The listing builds one solid part. Answer for the finished solid, in the listing's coordinates (mm). Give positions to 0.01 mm unless a question says otherwise; leave off trailing zeros. Write each loop counter-clockwise with the first axis right and the second up, starting at its lowest first coordinate (ties: lowest second). Pieces come first, ordered by that corner, then holes.
```python
from build123d import *

# Parameters (mm, degrees)
BOSS_EXTRUDE4_DEPTH                             = 4.5
CSK_FOR_M3_FLAT_HEAD_MACHINE_SCREW1_D           = 3.4
CSK_FOR_M3_FLAT_HEAD_MACHINE_SCREW1_CSINK_D     = 6.3
CSK_FOR_M3_FLAT_HEAD_MACHINE_SCREW1_CSINK_ANGLE = 90


with BuildPart() as part:
    # Sketch6 → Boss-Extrude4 (new body)
    with BuildSketch(Plane(origin=(0, 0, 0), x_dir=(1, 0, 0), z_dir=(0, 1, 0))):
        with BuildLine():
            Line((-37.735031535, 17.5893733), (-18.832983626, 28.967073503))
            ThreePointArc((-18.832983626, 28.967073503), (1.730983294, 34.678659015), (22.294950215, 28.967073503))
            Line((22.294950215, 28.967073503), (41.196998124, 17.5893733))
            Line((41.196998124, 17.5893733), (41.599351581, -4.469130473))
            ThreePointArc((41.599351581, -4.469130473), (1.730983294, -45.071340985), (-38.137384993, -4.469130473))
            Line((-38.137384993, -4.469130473), (-37.735031535, 17.5893733))
        make_face()
    extrude(amount=BOSS_EXTRUDE4_DEPTH)

    # CSK for M3 Flat Head Machine Screw1 (through all)
    with Locations(Plane(origin=(0, 0, 5.6), x_dir=(1, 0, 0), z_dir=(0, -1, 0))):
        with Locations((1.730983294, -6.903659015), (1.730983294, 6.096340985)):
            CounterSinkHole(CSK_FOR_M3_FLAT_HEAD_MACHINE_SCREW1_D / 2, CSK_FOR_M3_FLAT_HEAD_MACHINE_SCREW1_CSINK_D / 2, counter_sink_angle=CSK_FOR_M3_FLAT_HEAD_MACHINE_SCREW1_CSINK_ANGLE)


solid = part.part
```
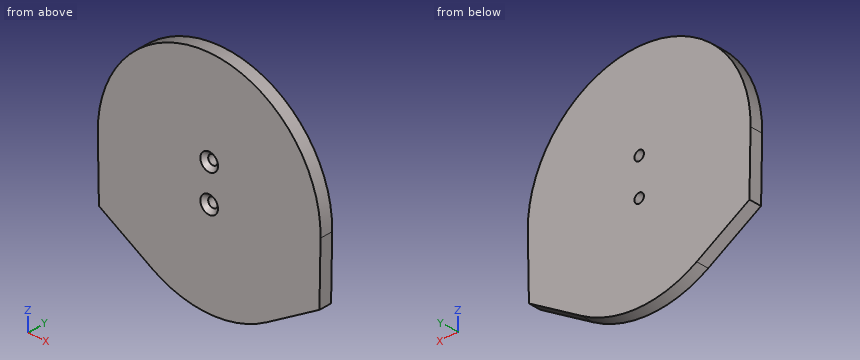
Item 1: A cutting plane is placed at A-A, the plane y = 2.35. Give the vertices of the cut face in (x, z) (3 decimals), plus the area to 3 significant figures.
Conclusion:
outline: (-38.137, 4.469) - (-37.735, -17.589) - (-18.833, -28.967) arc R39.875 ccw to (22.295, -28.967) - (41.197, -17.589) - (41.599, 4.469) arc R39.875 ccw (long way) to start; hole circle Ø3.4 at (1.731, -1.304); hole circle Ø3.4 at (1.731, 11.696)
area: 5,130 mm2
Item 2: Each of these flat-tipped pins is pushed along its axis until it touches: P1, Ø2.5, axis at x = 1.73, z = 11.7, coming from the +Y side; P2, Ø1.5, axis at x = 5, y = 2, coming from the -Z side. Where does it stop, or does it pass through?
Conclusion:
P1: passes through
P2: stops at z = -34.6
Item 3: Consider probe 1 along Z at (x, y) = (3, 4.3); probe 2 along Z at (x, y) = (2.5, 4.35); probe 3 along X at (y, z) = (0.7, -19). Determine where each line is inside the solid, lowest interval first.
Conclusion:
probe 1: z = -34.66 to -2.43, -0.17 to 10.57, 12.83 to 45.05
probe 2: z = -34.67 to -2.82, 0.21 to 10.18, 13.21 to 45.06
probe 3: x = -35.39 to 38.85
Item 4: A cutting plane is placed at C-C, the plane z = 31.5. Give the vertices of the cut face in (x, y).
Conclusion:
outline: (-28.24, 0) - (31.7, 0) - (31.7, 4.5) - (-28.24, 4.5) - close
Item 5: A cutting plane is placed at B-B, the plane x = 33.5. Give the vertices of the cut face in (y, z) (3 decimals).
Conclusion:
outline: (0, -22.222) - (4.5, -22.222) - (4.5, 29.295) - (0, 29.295) - close
